Source: CAD feature listing. Evaluate the final solid. Frame: model axes, mm. Face numbers are marked on the shaded views. Give positions to 0.01 mm unless a question says otherwise; leave off trailing zeros. Order: outer loops, then holes, each group sorted by start corner. A loop starts at its lowest first (then second) coordinate and runs counter-clockwise, first axis right, second up. Notation, with made-up numbers: M -3,87 L 17,87 A22 ccw 17,96 Z; hole C -21,75 d11. An arc over 180 degrees is marked long. Use CSV: the item, a comma, the result in double quotes. Start each with the question number.
Item 1: Section query D-D on x = 5.5. Return loops of the section in (y, z), and give its area (3 significant figures).
Item 2: Pull-direction query (X, two-part tool) for the marked faces 1, 2, 3 and 4; classes: +X half, -X half, draft (parallel to the pull), parting line (faces both ways), or undercut.
Item 3: Ray query, probe 1 along X at (y, z) = (14, -47) (3 decimals); probe 2 along Y at (x, z) = (13.55, 0) (3 decimals); probe 3 along Y at (x, z) = (-6, -51.5). Return the intervals inside material, ascending. Write a range as from..to.
Item 4: Section query B-B on z = -25.4. Return loops of the section in (x, y) (3 decimals).
Item 5: Section query A-A on y = 17. Return loops of the section in (x, z) (3 decimals), and give its area (3 significant figures).
Item 6: Section query C-C on z = 36. Return loops of the section in (x, y) (3 decimals).
Item 7: First-contact query: pin 1 (1.5 mm diameter, centred on x = 11.5, z = 39, fed in from -Y); pin 2 (1 mm diameter, centred on x = -9.5, z = -31.5, fed in from -Y). Flat tips, straight axial feed; report the tip coordinate or a pass-through.
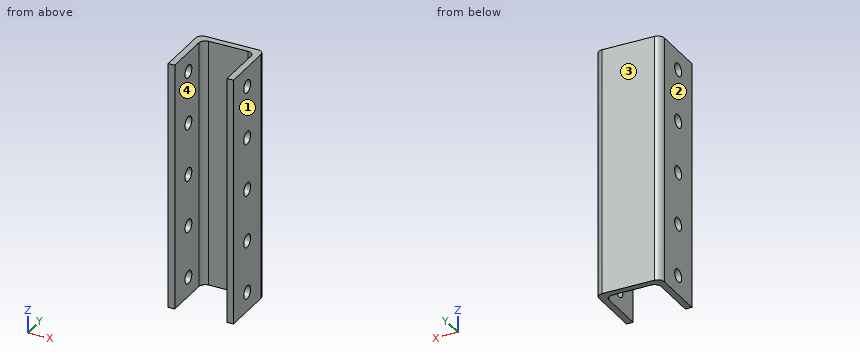
Autodesk Inventor part; units mm, degrees
ref_plane "YZ Plane" through (0, 0, 0) normal (1, 0, 0) x (0, 1, 0)
ref_plane "XZ Plane" through (0, 0, 0) normal (0, 1, 0) x (-1, 0, 0)
ref_plane "XY Plane" through (0, 0, 0) normal (0, 0, 1) x (1, 0, 0)
sketch "Sketch1" plane through (0, 0, 0) normal (0, 0, 1) x (1, 0, 0)
  line L0 (-15.875, 0) -> (-12.7, 0)
  line L1 (-12.7, 0) -> (-12.7, 22.352)
  line L2 (-9.525, 25.527) -> (9.525, 25.527)
  line L3 (12.7, 22.352) -> (12.7, 0)
  line L4 (12.7, 0) -> (15.875, 0)
  line L5 (15.875, 0) -> (15.875, 25.527)
  line L6 (12.7, 28.702) -> (-12.7, 28.702)
  line L7 (-15.875, 25.527) -> (-15.875, 0)
  arc A0 (-9.525, 25.527) -> (-12.7, 22.352) centre (-9.525, 22.352) ccw
  arc A1 (12.7, 22.352) -> (9.525, 25.527) centre (9.525, 22.352) ccw
  arc A2 (-12.7, 28.702) -> (-15.875, 25.527) centre (-12.7, 25.527) ccw
  arc A3 (15.875, 25.527) -> (12.7, 28.702) centre (12.7, 25.527) ccw
  line L8 (0, 35.2315) -> (0, -5.8719)
  point P0 (0, 0)
  dimension "d0" = 28.702
  dimension "d1" = 31.75
  dimension "d2" = 3.175
  dimension "d3" = 3.175
  dimension "d4" = 3.175
extrude "Extrusion1" add sketch "Sketch1" along normal mid plane 120.396
sketch "Sketch4" plane through (15.875, 0, 60.198) normal (1, 0, 0) x (0, 0, -1)
  line L0 (-79.375, 0) -> (476.25, 0)
  line L1 (60.198, -5.7404) -> (60.198, 34.4424)
  circle A0 centre (60.198, 12.7) radius 3.175
  point P0 (60.198, 0)
  dimension "d35" = 12.7
  dimension "d36" = 0
  dimension "d37" = 6.35
extrude "Extrusion4" cut sketch "Sketch4" against normal up to surface (31.75 mm away)
pattern_linear "Rectangular Pattern3" count 20 spacing 25.4 along (0, 0, 1) count 20 spacing 25.4 along (0, 0, -1) of "Extrusion4"
equation "\"d5\" = Support3Length"
equation "\"Support3Length\" = 120.396"
properties part number "NSupportChannel3" material "Aluminum 6061"
Verdict:
1,outline,"M 25.53,-60.2 L 28.7,-60.2 L 28.7,60.2 L 25.53,60.2 Z"
1,area,"382 mm2"
2,face 1,"+X half"
2,face 2,"-X half"
2,face 3,"draft"
2,face 4,"undercut"
3,probe 1,"-15.875..-12.7, 12.7..15.875"
3,probe 2,"0..9.525, 15.875..28.586"
3,probe 3,"25.53..28.7"
4,outline,"M -15.875,0 L -12.7,0 L -12.7,9.525 L -15.875,9.525 Z; M -15.875,15.875 L -12.7,15.875 L -12.7,22.352 A3.175 cw -9.525,25.527 L 9.525,25.527 A3.175 cw 12.7,22.352 L 12.7,15.875 L 15.875,15.875 L 15.875,25.527 A3.175 ccw 12.7,28.702 L -12.7,28.702 A3.175 ccw -15.875,25.527 Z; M 12.7,0 L 15.875,0 L 15.875,9.525 L 12.7,9.525 Z"
5,outline,"M -15.875,-60.198 L -12.7,-60.198 L -12.7,60.198 L -15.875,60.198 Z; M 12.7,-60.198 L 15.875,-60.198 L 15.875,60.198 L 12.7,60.198 Z"
5,area,"765 mm2"
6,outline,"M -15.875,0 L -12.7,0 L -12.7,22.352 A3.175 cw -9.525,25.527 L 9.525,25.527 A3.175 cw 12.7,22.352 L 12.7,0 L 15.875,0 L 15.875,25.527 A3.175 ccw 12.7,28.702 L -12.7,28.702 A3.175 ccw -15.875,25.527 Z"
7,pin 1,"y = 23.98"
7,pin 2,"y = 25.49"
